from build123d import *

# Parameters (mm, degrees)
SKETCH_1_W          = 40
SKETCH_1_H          = 20
EXTRUDE_1_DEPTH     = 6
SKETCH_2_W          = 40
SKETCH_2_H          = 32.5
EXTRUDE_2_DEPTH     = 35
CUT_EXTRUDE_1_DEPTH = 13
CUT_EXTRUDE_2_DEPTH = 2
SKETCH_6_W          = 40
SKETCH_6_H          = 41
CUT_EXTRUDE_3_DEPTH = 5
SKETCH_8_R          = 1.7
SKETCH_8_R_2        = 1.4
CUT_EXTRUDE_4_DEPTH = 49.79805324
CUT_EXTRUDE_5_REACH = 48.165
SKETCH_9_W          = 40
SKETCH_9_H          = 3
CHAMFER_1_SIZE2     = 6
CHAMFER_1_SIZE      = 0.8
CUT_EXTRUDE_6_REACH = 49.173
SKETCH_11_W         = 0.4
SKETCH_11_H         = 41


with BuildPart() as part:
    # Эскиз1 → Бобышка-Вытянуть1 (new body)
    with BuildSketch(Plane.XY):
        Rectangle(SKETCH_1_W, SKETCH_1_H)
    extrude(amount=EXTRUDE_1_DEPTH)

    # Эскиз2 → Бобышка-Вытянуть2 (add)
    with BuildSketch(Plane(origin=(0, 0, 0), x_dir=(-1, 0, 0), z_dir=(0, 0, -1))):
        with Locations((0, 6.25)):
            Rectangle(SKETCH_2_W, SKETCH_2_H)
    extrude(amount=EXTRUDE_2_DEPTH)

    # Эскиз3 → Вырез-Вытянуть1 (cut)
    with BuildSketch(Plane.XZ.offset(10)):
        Polygon((-7, 6), (-7, -1), (-8.6, -1), (-8.6, -18.5), (-4.5, -30.5), (-4.5, -34), (-3.5, -34), (-3.5, -35), (3.5, -35), (3.5, -34), (4.5, -34), (4.5, -30.5), (8.6, -18.5), (8.6, -1), (7, -1), (7, 6), align=None)
    extrude(amount=-CUT_EXTRUDE_1_DEPTH, mode=Mode.SUBTRACT)

    # Эскиз5 → Вырез-Вытянуть2 (cut)
    with BuildSketch(Plane.XZ.offset(-3)):
        Polygon((-8.6, -1), (8.6, -1), (8.6, -18.5), (4.5, -30.5), (4.5, -34), (-4.5, -34), (-4.5, -30.5), (-8.6, -18.5), align=None)
    extrude(amount=-CUT_EXTRUDE_2_DEPTH, mode=Mode.SUBTRACT)

    # Эскиз6 → Вырез-Вытянуть3 (cut)
    with BuildSketch(Plane.XZ.offset(10)):
        with Locations((0, -14.5)):
            Rectangle(SKETCH_6_W, SKETCH_6_H)
    extrude(amount=-CUT_EXTRUDE_3_DEPTH, mode=Mode.SUBTRACT)

    # Эскиз8 → Вырез-Вытянуть4 (cut, through all)
    with BuildSketch(Plane.XZ.offset(5)):
        with Locations((12, -30.5)):
            Circle(SKETCH_8_R)
        with Locations((14.3, -6)):
            Circle(SKETCH_8_R_2)
        with Locations(Location((-12, -30.5, 0), (0, 0, 180))):
            Circle(SKETCH_8_R)
        with Locations(Location((-14.3, -6, 0), (0, 0, 180))):
            Circle(SKETCH_8_R_2)
    extrude(amount=-CUT_EXTRUDE_4_DEPTH, mode=Mode.SUBTRACT)

    # Вырез-Вытянуть5: up to this face of the body (flat: up to its plane)
    cut_extrude_5_end = Plane(part.part.faces().sort_by_distance((0, 9.272988506, -35))[0])
    # Эскиз9 → Вырез-Вытянуть5 (cut, up to the picked face)
    with BuildSketch(Plane.XY, mode=Mode.PRIVATE) as cut_extrude_5_sk1:
        with Locations((0, 21)):
            Rectangle(SKETCH_9_W, SKETCH_9_H)
    cut_extrude_5_tool1 = split(extrude(cut_extrude_5_sk1.sketch, amount=-CUT_EXTRUDE_5_REACH, mode=Mode.PRIVATE), bisect_by=cut_extrude_5_end, keep=Keep.BOTH, mode=Mode.PRIVATE)
    add(cut_extrude_5_tool1.solids().sort_by(Axis((0, 21, 0), (0, 0, -1)))[0], mode=Mode.SUBTRACT)

    # Фаска1
    chamfer_1_edges = [part.edges().sort_by_distance(p)[0] for p in [
        (0, 10, 6),
    ]]
    chamfer_1_side = [part.faces().sort_by_distance(p)[0] for p in [
        (0, 9.984, 6),
    ]]
    chamfer(chamfer_1_edges, length=CHAMFER_1_SIZE - 0.0001, length2=CHAMFER_1_SIZE2 - 0.0001, reference=chamfer_1_side[0])  # a hair under: the kernel refuses the full size

    # Вырез-Вытянуть6: up to this face of the body (flat: up to its plane)
    cut_extrude_6_end = Plane(part.part.faces().sort_by_distance((13.552984989, -5, -15.226398396))[0])
    # Эскиз11 → Вырез-Вытянуть6 (cut, up to the picked face)
    with BuildSketch(Plane(origin=(0, 19.5, 0), x_dir=(1, 0, 0), z_dir=(0, 1, 0)), mode=Mode.PRIVATE) as cut_extrude_6_sk1:
        with Locations((-19.8, 14.5)):
            Rectangle(SKETCH_11_W, SKETCH_11_H)
    cut_extrude_6_tool1 = split(extrude(cut_extrude_6_sk1.sketch, amount=-CUT_EXTRUDE_6_REACH, mode=Mode.PRIVATE), bisect_by=cut_extrude_6_end, keep=Keep.BOTH, mode=Mode.PRIVATE)
    # Эскиз11 → Вырез-Вытянуть6 (cut, up to the picked face)
    with BuildSketch(Plane(origin=(0, 19.5, 0), x_dir=(1, 0, 0), z_dir=(0, 1, 0)), mode=Mode.PRIVATE) as cut_extrude_6_sk2:
        with Locations((19.8, 14.5)):
            Rectangle(SKETCH_11_W, SKETCH_11_H)
    cut_extrude_6_tool2 = split(extrude(cut_extrude_6_sk2.sketch, amount=-CUT_EXTRUDE_6_REACH, mode=Mode.PRIVATE), bisect_by=cut_extrude_6_end, keep=Keep.BOTH, mode=Mode.PRIVATE)
    add(cut_extrude_6_tool1.solids().sort_by(Axis((-19.8, 19.5, -14.5), (0, -1, 0)))[0], mode=Mode.SUBTRACT)
    add(cut_extrude_6_tool2.solids().sort_by(Axis((19.8, 19.5, -14.5), (0, -1, 0)))[0], mode=Mode.SUBTRACT)


solid = part.part
The model under review builds one solid part; all positions refer to its coordinate system, in mm. A direction names the side the tool comes from. Give positions to 0.01 mm unless a question says otherwise; leave off trailing zeros. Order: outer loops, then holes, each group sorted by start corner. A loop starts at its lowest first (then second) coordinate and runs counter-clockwise, first axis right, second up. Notation, with made-up numbers: (59.5, -3) -> (68.5, -3) arc R27 ccw to (68.5, 18) -> close; hole circle Ø8 at (20.5, -11.75). An arc over 180 degrees is marked (long way). Write item = value, one per line. Start each with the question number.
(1) Take a section at D-D (y = 5.75). Write out the cut boundary in (x, z).
(2) For L1, parallel to X at y = 16.25, z = -32; L2, parallel to Z at x = 14.3, y = 10.5; L3, parallel to Y at x = -3, z = -26, list the stretches that pass through material, from the lowest coordinate up. Write a range as from..to.
(3) Draft analysis for pull direction X (two halves, no side actions). For faces 4 (the flat face through (19.6, 7, -14)), 5 (the flat face through (0, 3, 3)), 6 (the flat face through (0, 15, 0)), state which applies: +X half, -X half, draft (parallel to the pull), parting line (faces both ways), or undercut.
(4) For pin 1 Ø0.8 at (x, z) = (-0.5, -34.5) entering from -Y, flat-tipped, find the tip position at first contact; note if it passes through.
(5) Tool access review of faces 1 (the cylindrical face through (-15.635, 7.078, -6.421)), 2 (the flat face through (7, -1, 2)), 3 (the flat face through (0.1, 3.3, -1)): name each direction out of +Z, -Z, +X, -X, +Y, -Y from which nothing blocks a thin tool from reaching the whole face with its end or side.
(6) Take a section at A-A (y = -0.75). Write out the cut boundary in (x, z).
(7) Take a section at C-C (z = -6). Write out the cut boundary in (x, y).
Returned:
q1.outline = (-19.6, -35) -> (19.6, -35) -> (19.6, 6) -> (-19.6, 6) -> close; hole circle Ø2.8 at (-14.3, -6); hole circle Ø3.4 at (-12, -30.5); hole circle Ø3.4 at (12, -30.5); hole circle Ø2.8 at (14.3, -6)
q2.L1 = -19.6..-12.8, -11.2..11.2, 12.8..19.6
q2.L2 = -35..-7.4, -4.6..0
q2.L3 = 5..19.5
q3.face_4 = +X half
q3.face_5 = undercut
q3.face_6 = draft
q4.pin_1 = 3
q5.face_1 = +Y, -Y
q5.face_2 = +Z, -Y
q5.face_3 = -Y
q6.outline = (-19.6, -35) -> (-3.5, -35) -> (-3.5, -34) -> (-4.5, -34) -> (-4.5, -30.5) -> (-8.6, -18.5) -> (-8.6, -1) -> (-7, -1) -> (-7, 6) -> (-19.6, 6) -> close; (3.5, -35) -> (19.6, -35) -> (19.6, 6) -> (7, 6) -> (7, -1) -> (8.6, -1) -> (8.6, -18.5) -> (4.5, -30.5) -> (4.5, -34) -> (3.5, -34) -> close; hole circle Ø2.8 at (-14.3, -6); hole circle Ø3.4 at (-12, -30.5); hole circle Ø3.4 at (12, -30.5); hole circle Ø2.8 at (14.3, -6)
q7.outline = (-19.6, -5) -> (-15.7, -5) -> (-15.7, 19.5) -> (-19.6, 19.5) -> close; (-12.9, -5) -> (-8.6, -5) -> (-8.6, 5) -> (8.6, 5) -> (8.6, -5) -> (12.9, -5) -> (12.9, 19.5) -> (-12.9, 19.5) -> close; (15.7, -5) -> (19.6, -5) -> (19.6, 19.5) -> (15.7, 19.5) -> close
